Answer from the drawing. Dimensions are ordinates in mm from the lowest x, y and z of the part. A direction names the side the tool comes from. Give positions to 0.01 mm unless a question says otherwise; leave off trailing zeros. Write each loop counter-clockwise with the first axis right and the second up, starting at its lowest first coordinate (ties: lowest second). Pieces come first, ordered by that corner, then holes. Notation, with made-up numbers: M 9.25,-13 L 33.25,-13 A29 cw 33.25,11 Z; hole C -4,8.25 d1. An arc over 180 degrees is marked long. Answer as a JSON object with one key per item and string values.
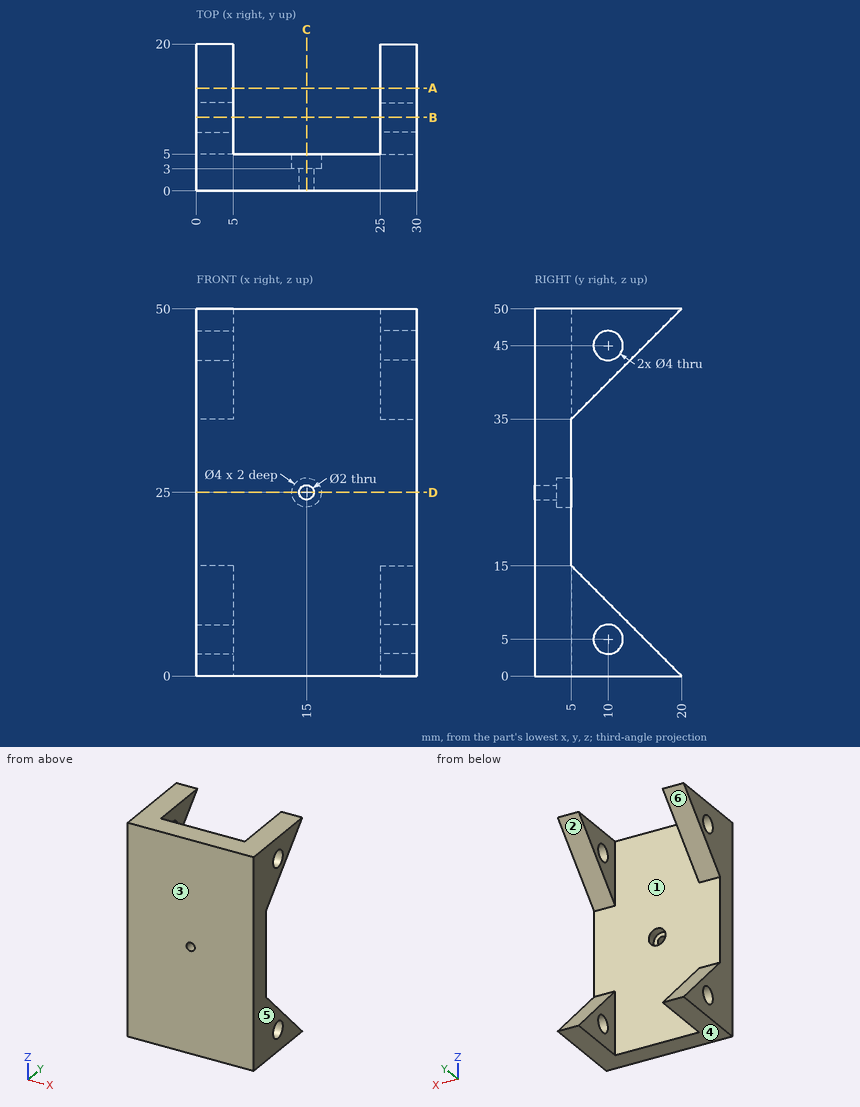
1. A flat-ended cylindrical pin translates along its axis: pin 1 (4 mm diameter, centred on x = 5, z = 21, fed in from +Y). Find the tip coordinate at first contact, or state that the pin passes through.
Verdict:
{"pin 1": "stops at y = 5"}
2. A cutting plane is placed at A-A, the plane y = 14. Give the vertices of the cut face in (x, z).
Verdict:
{"outline": "M 0,0 L 5,0 L 5,6 L 0,6 Z; M 0,44 L 5,44 L 5,50 L 0,50 Z; M 25,0 L 30,0 L 30,6 L 25,6 Z; M 25,44 L 30,44 L 30,50 L 25,50 Z"}
3. A cutting plane is placed at C-C, the plane x = 15. Give the vertices of the cut face in (y, z), plus the area to 3 significant figures.
Verdict:
{"outline": "M 0,0 L 5,0 L 5,23 L 3,23 L 3,24 L 0,24 Z; M 0,26 L 3,26 L 3,27 L 5,27 L 5,50 L 0,50 Z", "area": "236 mm2"}
4. A cutting plane is placed at D-D, the plane z = 25. Give the vertices of the cut face in (x, y).
Verdict:
{"outline": "M 0,0 L 14,0 L 14,3 L 13,3 L 13,5 L 0,5 Z; M 16,0 L 30,0 L 30,5 L 17,5 L 17,3 L 16,3 Z"}
5. A cutting plane is placed at B-B, the plane y = 10. Count the separate pieces of the cut face and the enclosed holes in it, plus the area to 3 significant figures.
Verdict:
{"separate pieces": "8", "enclosed holes": "0", "area": "120 mm2"}
6. For the marked faces 1, 2 and 3, determine the directions among +Z, -Z, +X, -X, +Y, -Y from which every point of the face is accessible in a straight line to the end or side of a thin tool.
Verdict:
{"face 1": "+Y", "face 2": "+X, -X, +Y", "face 3": "+Z, -Z, +X, -X, -Y"}
7. Consider line 1 along Z through (x, y) = (3.95, 10); line 2 along Y through (x, z) = (18.75, 11.5); line 3 along X through (y, z) = (16, 47). Determine where each line is inside the solid, lowest interval first.
Verdict:
{"line 1": "z = 0 to 3, 7 to 10, 40 to 43, 47 to 50", "line 2": "y = 0 to 5", "line 3": "x = 0 to 5, 25 to 30"}
8. The mould has two halves that part along Z. Classify the marked faces 4, 5 and 6: released by +Z, released by -Z, zero draft, split by the parting line, or undercut.
Verdict:
{"face 4": "released by -Z", "face 5": "zero draft", "face 6": "undercut"}
